Work out the finished part from the listing and answer in its coordinate system (mm). A direction names the side the tool comes from. Give positions to 0.01 mm unless a question says otherwise; leave off trailing zeros. Order: outer loops, then holes, each group sorted by start corner. A loop starts at its lowest first (then second) coordinate and runs counter-clockwise, first axis right, second up.
```python
from build123d import *

# Parameters (mm, degrees)
SKETCH1_W                = 50
SKETCH1_H                = 23
BOSS_EXTRUDE1_DEPTH      = 1
FILLET1_R                = 1
BOSS_EXTRUDE2_DEPTH      = 1.5
BOSS_EXTRUDE2_DEPTH_BACK = 5.5
SKETCH3_W                = 8
SKETCH3_H                = 6
BOSS_EXTRUDE3_DEPTH      = 5.5


with BuildPart() as part:
    # Sketch1 → Boss-Extrude1 (new body)
    with BuildSketch(Plane(origin=(0, 0, 0), x_dir=(1, 0, 0), z_dir=(0, 1, 0))):
        with Locations((25, 11.5)):
            Rectangle(SKETCH1_W, SKETCH1_H)
    extrude(amount=BOSS_EXTRUDE1_DEPTH)

    # Fillet1
    fillet1_edges = [part.edges().sort_by_distance(p)[0] for p in [
        (0, 0.5, -23),
        (50, 0.5, -23),
        (50, 0.5, 0),
        (0, 0.5, 0),
    ]]
    fillet(fillet1_edges, radius=FILLET1_R)

    # Sketch2 → Boss-Extrude2 (add, two sides: drawn at the far end of the back side and taken through both)
    with BuildSketch(Plane.ZY.offset(-BOSS_EXTRUDE2_DEPTH_BACK)):
        with BuildLine():
            Line((-8.5, 1), (-14.5, 1))
            ThreePointArc((-14.5, 1), (-16, 2.5), (-14.5, 4))
            Line((-14.5, 4), (-8.5, 4))
            ThreePointArc((-8.5, 4), (-7, 2.5), (-8.5, 1))
        make_face()
    extrude(amount=BOSS_EXTRUDE2_DEPTH + BOSS_EXTRUDE2_DEPTH_BACK)

    # Sketch3 → Boss-Extrude3 (add)
    with BuildSketch(Plane(origin=(0, 1, 0), x_dir=(1, 0, 0), z_dir=(0, 1, 0))):
        with Locations((11, 20)):
            Rectangle(SKETCH3_W, SKETCH3_H)
    extrude(amount=BOSS_EXTRUDE3_DEPTH)


solid = part.part
```
1. Straight lines are drawn through the part: probe 1 along X at (y, z) = (2.75, -19.25); probe 2 along Z at (x, y) = (11, 5); probe 3 along Y at (x, z) = (42, -8.25). For each, find the intervals that lie inside material, in ascending order.
Findings below:
probe 1: x = 7 to 15
probe 2: z = -23 to -17
probe 3: y = 0 to 1
2. The part is cut by section C-C (x = 4.5). Write down the section's boundary in (y, z), then the cut area to 3 significant figures.
Findings below:
outline: (0, -23) - (1, -23) - (1, -14.5) arc R1.5 ccw to (4, -14.5) - (4, -8.5) arc R1.5 ccw to (1, -8.5) - (1, 0) - (0, 0) - close
area: 48.1 mm2
3. The part is cut by section D-D (y = 4.75). Write down the section's boundary in (x, z).
Findings below:
outline: (7, -23) - (15, -23) - (15, -17) - (7, -17) - close
4. Which of the six approach directions +Z, -Z, +X, -X, +Y, -Y give full straight-line access (tool end or side, diameter ignored) to faces 1 (the face through (-1, 1, -11)), 2 (the face through (11, 4, -17)), 3 (the face through (5.5, 3, -11))?
Findings below:
face 1: +Z, -Z, -X, -Y
face 2: +Z, +X, -X, +Y
face 3: +Z, -Z, +X, +Y
5. Given P1, Ø6.5, axis at x = 2.5, z = -11, coming from the +Y side; P2, Ø1.5, axis at y = 3, z = -12, coming from the +X side; P3, Ø3, axis at x = 12.5, y = 4.5, coming from the +Z side, each flat-ended and moving along its own axis, determine where each tip first touches the part or whether it passes through.
Findings below:
P1: stops at y = 4
P2: stops at x = 5.5
P3: stops at z = -17
6. The part is cut by section B-B (z = -18.75). Write down the section's boundary in (x, y), then the cut area to 3 significant figures.
Findings below:
outline: (0, 0) - (50, 0) - (50, 1) - (15, 1) - (15, 6.5) - (7, 6.5) - (7, 1) - (0, 1) - close
area: 94.0 mm2
7. The part is cut by section A-A (y = 2.5). Write down the section's boundary in (x, z).
Findings below:
outline: (-1.5, -16) - (5.5, -16) - (5.5, -7) - (-1.5, -7) - close; (7, -23) - (15, -23) - (15, -17) - (7, -17) - close
